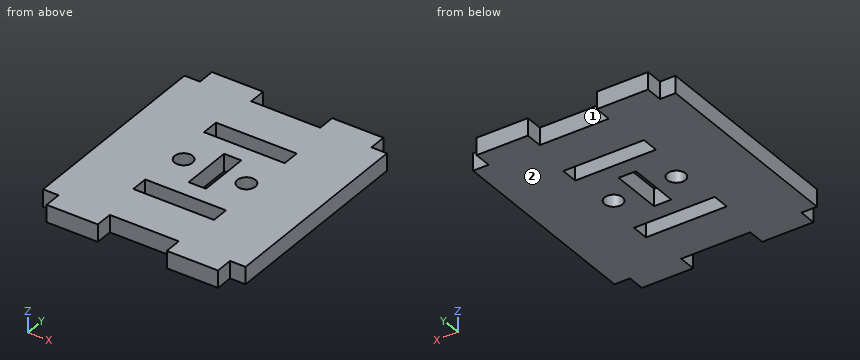
Autodesk Inventor part; units mm, degrees
ref_plane "YZ Plane" through (0, 0, 0) normal (1, 0, 0) x (0, 1, 0)
ref_plane "XZ Plane" through (0, 0, 0) normal (0, 1, 0) x (-1, 0, 0)
ref_plane "XY Plane" through (0, 0, 0) normal (0, 0, 1) x (1, 0, 0)
sketch "Sketch1" plane through (0, 0, 0) normal (0, 0, 1) x (1, 0, 0)
  line L0 (-37.5, 37.9177) -> (-31.7388, 37.9177)
  line L1 (37.5, 37.9177) -> (37.5, -37.9177)
  line L2 (37.5, -37.9177) -> (31.7388, -37.9177)
  line L3 (-37.5, -37.9177) -> (-37.5, 37.9177)
  line L4 (-31.7388, 37.9177) -> (-31.7388, 44.3077)
  line L5 (-31.7388, 44.3077) -> (-12.78, 44.3077)
  line L6 (-12.78, 44.3077) -> (-12.78, 37.9177)
  line L7 (0, 37.9177) -> (0, -37.9177) construction
  line L8 (-37.5, 0) -> (37.5, 0) construction
  line L9 (-12.78, 37.9177) -> (12.78, 37.9177)
  line L10 (31.7388, 37.9177) -> (31.7388, 44.3077)
  line L11 (31.7388, 44.3077) -> (12.78, 44.3077)
  line L12 (12.78, 44.3077) -> (12.78, 37.9177)
  line L13 (-31.7388, -37.9177) -> (-31.7388, -44.3077)
  line L14 (-31.7388, -44.3077) -> (-12.78, -44.3077)
  line L15 (-12.78, -44.3077) -> (-12.78, -37.9177)
  line L16 (12.78, -44.3077) -> (12.78, -37.9177)
  line L17 (31.7388, -44.3077) -> (12.78, -44.3077)
  line L18 (31.7388, -37.9177) -> (31.7388, -44.3077)
  line L19 (31.7388, 37.9177) -> (37.5, 37.9177)
  line L20 (-31.7388, -37.9177) -> (-37.5, -37.9177)
  line L21 (12.78, -37.9177) -> (-12.78, -37.9177)
  line L22 (-14.945, 15.7638) -> (14.945, 15.7638)
  line L23 (14.945, 15.7638) -> (14.945, 22.1538)
  line L24 (14.945, 22.1538) -> (-14.945, 22.1538)
  line L25 (-14.945, 22.1538) -> (-14.945, 15.7638)
  line L26 (-14.945, -15.7638) -> (14.945, -15.7638)
  line L27 (14.945, -15.7638) -> (14.945, -22.1538)
  line L28 (14.945, -22.1538) -> (-14.945, -22.1538)
  line L29 (-14.945, -22.1538) -> (-14.945, -15.7638)
  line L30 (-3.195, 9.4794) -> (3.195, 9.4794)
  line L31 (3.195, 9.4794) -> (3.195, -9.4794)
  line L32 (3.195, -9.4794) -> (-3.195, -9.4794)
  line L33 (-3.195, -9.4794) -> (-3.195, 9.4794)
  line L34 (-14.945, 18.9588) -> (14.945, 18.9588) construction
  circle A0 centre (-11.6112, 0) radius 3.3338
  circle A1 centre (11.6112, 0) radius 3.3338
  point P0 (0, 0)
  point P1 (0, 22.1538)
  point P2 (3.195, 0)
  point P3 (0, 0)
  point P4 (0, 9.4794)
  point P5 (0, 0)
  point P6 (-22.2594, -44.3077)
  dimension "d0" = 75
  dimension "d1" = 75.8353
  dimension "d2" = 18.9588
  dimension "d3" = 6.39
  dimension "d4" = 12.78
  dimension "d21" = 6.39
  dimension "d22" = 29.89
  dimension "d24" = 18.9588
  dimension "d25" = 6.39
  dimension "d30" = 37.9177
  dimension "d41" = 6.6675
extrude "Extrusion4" add sketch "Sketch1" along normal blind 6.39
equation "\"d1\" = DiskGap"
equation "\"d2\" = 0.25 * DiskGap"
equation "\"d3\" = WoodThickness"
equation "\"d4\" = 2 * WoodThickness"
equation "\"d21\" = WoodThickness"
equation "\"d22\" = 0.5 * ColumnWidth"
equation "\"d24\" = 0.25 * DiskGap"
equation "\"d25\" = WoodThickness"
equation "\"d30\" = 0.5 * DiskGap"
equation "\"d42\" = WoodThickness"
properties part number "LightDiskSupport" material "MDF Medium Density Fiberboard"
Here's how the part is built. I have some questions about the finished solid (model axes, mm). Face numbers are marked on the shaded views. Coordinates: 2 decimals unless noted, no trailing zeros. Write each loop counter-clockwise with the first axis right and the second up, starting at its lowest first coordinate (ties: lowest second). Pieces come first, ordered by that corner, then holes.
1) I'm going to push flat-ended pins straight in: pin 1 (1.9 mm diameter, centred on y = -40.5, z = 4.5, fed in from -X); pin 2 (1.7 mm diameter, centred on x = 34.5, z = 2.5, fed in from +Y); pin 3 (3 mm diameter, centred on x = -5, z = 2.5, fed in from -Y); pin 4 (4 mm diameter, centred on x = 11.61, y = 0, fed in from +Z). Where does each tip first touch, or does it pass through?
Filled in:
pin 1: stops at x = -31.74
pin 2: stops at y = 37.92
pin 3: stops at y = -37.92
pin 4: passes through
2) If we section it at D-D (y = 0): List the corners of the cut face in (x, z) for me (3 decimals), plus the area to 3 significant figures.
Filled in:
outline: (-37.5, 0) - (-14.945, 0) - (-14.945, 6.39) - (-37.5, 6.39) - close; (-8.277, 0) - (-3.195, 0) - (-3.195, 6.39) - (-8.277, 6.39) - close; (3.195, 0) - (8.277, 0) - (8.277, 6.39) - (3.195, 6.39) - close; (14.945, 0) - (37.5, 0) - (37.5, 6.39) - (14.945, 6.39) - close
area: 353 mm2
3) Thinking about a two-plate mould opening in X: for the marked faces 1 and 2, which applies, +X half, -X half, draft (parallel to the pull), parting line (faces both ways), or undercut?
Filled in:
face 1: undercut
face 2: draft
4) If we section it at B-B (x = 1): List the corners of the cut face in (y, z) for me.
Filled in:
outline: (-37.92, 0) - (-22.15, 0) - (-22.15, 6.39) - (-37.92, 6.39) - close; (-15.76, 0) - (-9.48, 0) - (-9.48, 6.39) - (-15.76, 6.39) - close; (9.48, 0) - (15.76, 0) - (15.76, 6.39) - (9.48, 6.39) - close; (22.15, 0) - (37.92, 0) - (37.92, 6.39) - (22.15, 6.39) - close
5) If I drill on line 1 (Y direction, x = 11.5, z = 4.25); line 2 (Y direction, x = -5.5, z = 5.25); line 3 (Y direction, x = -1.5, z = 4.75), over which ranges is the centre line in solid material (lowest first)?
Filled in:
line 1: y = -37.92 to -22.15, -15.76 to -3.33, 3.33 to 15.76, 22.15 to 37.92
line 2: y = -37.92 to -22.15, -15.76 to 15.76, 22.15 to 37.92
line 3: y = -37.92 to -22.15, -15.76 to -9.48, 9.48 to 15.76, 22.15 to 37.92
6) If we section it at C-C (z = 5): Count the separate pieces of the cut face and the enclosed holes in it, plus the area to 3 significant figures.
Filled in:
separate pieces: 1
enclosed holes: 5
area: 5,600 mm2
7) If we section it at A-A (y = -19): List the corners of the cut face in (x, z) for me (3 decimals).
Filled in:
outline: (-37.5, 0) - (-14.945, 0) - (-14.945, 6.39) - (-37.5, 6.39) - close; (14.945, 0) - (37.5, 0) - (37.5, 6.39) - (14.945, 6.39) - close
